The listing builds one solid part. Answer for the finished solid, in the listing's coordinates (mm). A direction names the side the tool comes from. Coordinates: 2 decimals unless noted, no trailing zeros. Order: outer loops, then holes, each group sorted by start corner. A loop starts at its lowest first (then second) coordinate and runs counter-clockwise, first axis right, second up. Notation, with made-up numbers: (-36.75, 10) - (-17.75, 10) arc R21 ccw to (-17.75, 47) - close; hole circle Ø4 at (43.5, 46). An arc over 180 degrees is marked (long way). One line per item, written item: value. Start each with the question number.
```python
from build123d import *

# Parameters (mm, degrees)
F1_DEPTH = 16
F2_DEPTH = 1


with BuildPart() as f1:
    # F0 (on Top) → F1 (new body)
    with BuildSketch(Plane.XY):
        Polygon((-46.304833, 19.758051), (-46.163612, -17.241679), (45.044052, -17.241949), (45.044052, 19.758051), align=None)
    extrude(amount=F1_DEPTH)

    # F0 (on Top) → F2 (join)
    with BuildSketch(Plane.XY):
        Polygon((46.859896, 21.758051), (-48.0788, 21.758051), (-47.923417, -18.952159), (46.859896, -18.952159), align=None)
        Polygon((45.044052, -17.241949), (-46.163612, -17.241679), (-46.304833, 19.758051), (45.044052, 19.758051), align=None, mode=Mode.SUBTRACT)
    extrude(amount=F2_DEPTH)


solid = f1.part
```
(1) The part is cut by section A-A on y = 3.5. Determine the outline of the cut face in (x, z), plus the area to 3 significant figures.
(2) The part is cut by section C-C on z = 15. Determine the outline of the cut face in (x, y).
(3) Flat-ended cylindrical pins translate along their axes: pin 1 Ø1 at (x, z) = (11, 13.5) entering from +Y; pin 2 Ø8 at (x, z) = (-24.5, 8) entering from -Y; pin 3 Ø1.5 at (y, z) = (-5, 7.5) entering from +X. Find the tip coordinate at first contact, or state that the pin passes through.
(4) Consider probe 1 along X at (y, z) = (-14.5, 13.75); probe 2 along Y at (x, z) = (2, 11.75); probe 3 along X at (y, z) = (17.5, 14). Determine where each line is inside the solid, lowest interval first.
(5) For faces 1 (the face through (0, 19.758, 8)), 2 (the face through (45.044, 1, 8)), 3 (the face through (-1, 2, 0)), determine the directions among +Z, -Z, +X, -X, +Y, -Y from which every point of the face is accessible in a straight line to the end or side of a thin tool.
(6) The part is cut by section B-B on x = 4. Determine the outline of the cut face in (y, z), plus the area to 3 significant figures.
Completed:
1. outline: (-48.01, 0) - (46.86, 0) - (46.86, 1) - (45.04, 1) - (45.04, 16) - (-46.24, 16) - (-46.24, 1) - (-48.01, 1) - close
1. area: 1,460 mm2
2. outline: (-46.3, 19.76) - (-46.16, -17.24) - (45.04, -17.24) - (45.04, 19.76) - close
3. pin 1: stops at y = 19.76
3. pin 2: stops at y = -17.24
3. pin 3: stops at x = 45.04
4. probe 1: x = -46.17 to 45.04
4. probe 2: y = -17.24 to 19.76
4. probe 3: x = -46.3 to 45.04
5. face 1: +Z, +X, -X, +Y
5. face 2: +Z, +X, +Y, -Y
5. face 3: -Z, +X, -X, +Y, -Y
6. outline: (-18.95, 0) - (21.76, 0) - (21.76, 1) - (19.76, 1) - (19.76, 16) - (-17.24, 16) - (-17.24, 1) - (-18.95, 1) - close
6. area: 596 mm2
